The listing builds one solid part. Answer for the finished solid, in the listing's coordinates (mm). Face numbers are marked on the shaded views. A direction names the side the tool comes from. Coordinates: 2 decimals unless noted, no trailing zeros. Loops run counter-clockwise (first coordinate to the right, second up) from the corner with the lowest first, then second, coordinate; pieces in that order, holes last. Notation, with made-up numbers: M -13.75,-11 L 21.25,-11 A18 cw 21.25,-1 Z; hole C 62.25,6 d10. An arc over 180 degrees is marked long. Answer as a JSON object with one key per item and string values. Group by question number.
1. Straight lines are drawn through the part: L1, parallel to Y at x = -4.5, z = 73; L2, parallel to X at y = -5, z = 80; L3, parallel to Z at x = -8.5, y = -12. For each, find the intervals that lie inside material, in ascending order.
2. A cutting plane is placed at B-B on x = -4. Give the vertices of the cut face in (y, z), and give its area (3 significant figures).
3. A cutting plane is placed at C-C on y = -3. Give the vertices of the cut face in (x, z).
4. For the marked faces 1, 2, 3 and 4, determine the directions among +Z, -Z, +X, -X, +Y, -Y from which every point of the face is accessible in a straight line to the end or side of a thin tool.
5. Given pin 1 (4 mm diameter, centred on x = 20.5, z = 95.5, fed in from -Y); pin 2 (12 mm diameter, centred on x = -4.5, z = 38, fed in from -Y); pin 3 (18 mm diameter, centred on x = 1.5, y = -53.5, fed in from -Z), each flat-ended and moving along its own axis, determine where each tip first touches the part or whether it passes through.
6. A cutting plane is placed at A-A on z = 101.5. Give the vertices of the cut face in (x, y), and give its area (3 significant figures).
7. A cutting plane is placed at D-D on x = 9. Give the vertices of the cut face in (y, z).
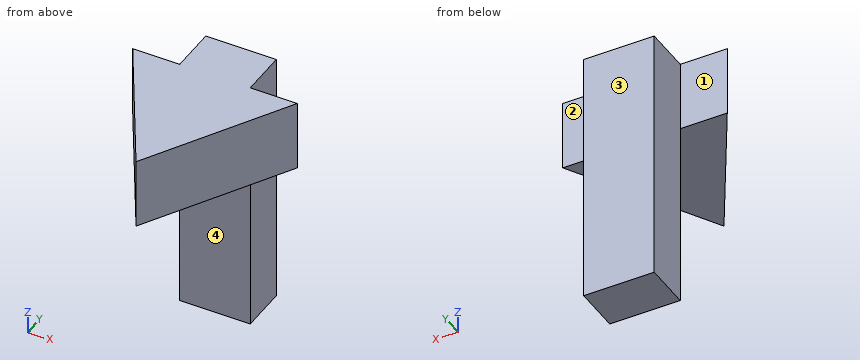
from build123d import *

# Parameters (mm, degrees)
F0_W     = 30
F0_H     = 20
F3_DEPTH = 110
F4_DEPTH = 30


with BuildPart() as f3:
    # F0 (on Top) → F3 (new body)
    with BuildSketch(Plane.XY):
        with Locations((1.746466, 0)):
            Rectangle(F0_W, F0_H)
    extrude(amount=F3_DEPTH)

    # F2 (on offset) → F4 (join)
    with BuildSketch(Plane.XY.offset(110)):
        Polygon((16.746466, -10), (-13.253534, -10), (-33.253534, -10), (1.746466, -70.621778), (36.746466, -10), align=None)
    extrude(amount=-F4_DEPTH)


solid = f3.part
From the geometry:
{
 "1": {"L1": "y = -10 to 10", "L2": "x = -13.25 to 16.75", "L3": "z = 80 to 110"},
 "2": {"outline": "M -60.67,80 L -10,80 L -10,0 L 10,0 L 10,110 L -60.67,110 Z", "area": "3,720 mm²"},
 "3": {"outline": "M -13.25,0 L 16.75,0 L 16.75,110 L -13.25,110 Z"},
 "4": {"face 1": "+Z, -Z, -X, +Y", "face 2": "+Z, -Z, +X, +Y", "face 3": "+Z, -Z, +X, -X, +Y", "face 4": "-Z, +X, -X, -Y"},
 "5": {"pin 1": "stops at y = -41.6", "pin 2": "stops at y = -10", "pin 3": "stops at z = 80"},
 "6": {"outline": "M -33.25,-10 L 1.75,-70.62 L 36.75,-10 L 16.75,-10 L 16.75,10 L -13.25,10 L -13.25,-10 Z", "area": "2,720 mm²"},
 "7": {"outline": "M -58.06,80 L -10,80 L -10,0 L 10,0 L 10,110 L -58.06,110 Z"}
}
